```python
from build123d import *

# Parameters (mm, degrees)
IZIM1_R                     = 4
Y_KSEKLIK_EKSTR_ZYON1_DEPTH = 16
IZIM2_W                     = 25
IZIM2_H                     = 6
KES_EKSTR_ZYON1_DEPTH       = 35
KES_EKSTR_ZYON2_DEPTH       = 36
KES_EKSTR_ZYON2_DEPTH_BACK  = 20
IZIM3_R                     = 3
SKETCH2_W                   = 46.387108154
SKETCH2_H                   = 28.761742624
CUT_EXTRUDE1_DEPTH          = 2
FILLET1_R                   = 5


with BuildPart() as part:
    # Çizim1 → Yükseklik-Ekstrüzyon1 (new body)
    with BuildSketch(Plane.XY):
        Polygon((-12.5, 28), (-12.5, -7), (12.5, -7), (12.5, 28), (12.5, 53), (6, 53), (4.5, 53), (4.5, 33), (-4.5, 33), (-4.5, 53), (-6, 53), (-12.5, 53), align=None)
        with Locations((0, 21)):
            Circle(IZIM1_R, mode=Mode.SUBTRACT)
        Circle(IZIM1_R, mode=Mode.SUBTRACT)
    extrude(amount=Y_KSEKLIK_EKSTR_ZYON1_DEPTH)

    # Çizim2 → Kes-Ekstrüzyon1 (cut)
    with BuildSketch(Plane.XZ.offset(7)):
        with Locations((0, 8)):
            Rectangle(IZIM2_W, IZIM2_H)
    extrude(amount=-KES_EKSTR_ZYON1_DEPTH, mode=Mode.SUBTRACT)

    # Çizim3 → Kes-Ekstrüzyon2 (cut, two sides: drawn at the far end of the back side and taken through both)
    with BuildSketch(Plane.ZY.offset(-4.5).offset(-KES_EKSTR_ZYON2_DEPTH_BACK)):
        with Locations(Location((8, 43, 0), (0, 0, 180))):
            Circle(IZIM3_R)
    extrude(amount=KES_EKSTR_ZYON2_DEPTH + KES_EKSTR_ZYON2_DEPTH_BACK, mode=Mode.SUBTRACT)

    # Sketch2 → Cut-Extrude1 (cut)
    with BuildSketch(Plane(origin=(0, 53, 0), x_dir=(1, 0, 0), z_dir=(0, 1, 0))):
        with Locations((-0.016890664, -9.346912489)):
            Rectangle(SKETCH2_W, SKETCH2_H)
    extrude(amount=-CUT_EXTRUDE1_DEPTH, mode=Mode.SUBTRACT)

    # Fillet1
    fillet1_edges = [part.edges().sort_by_distance(p)[0] for p in [
        (8.5, 51, 16),
        (-8.5, 51, 16),
        (8.5, 51, 0),
        (-8.5, 51, 0),
    ]]
    fillet(fillet1_edges, radius=FILLET1_R)


solid = part.part
```
Geometry check sheet. Reference: the model listing, model coordinates, mm. A direction names the side the tool comes from. Give positions to 0.01 mm unless a question says otherwise; leave off trailing zeros. Write each loop counter-clockwise with the first axis right and the second up, starting at its lowest first coordinate (ties: lowest second). Pieces come first, ordered by that corner, then holes. Notation, with made-up numbers: (-21.75, 85) -> (8.25, 85) arc R18 cw to (8.25, 111) -> close; hole circle Ø9 at (16.5, 16). An arc over 180 degrees is marked (long way). Use one line per item in the form item = value.
Item 1: Depth check by flat-ended pin: pin 1 Ø1.8 at (x, z) = (0, 7.5) entering from -Y; pin 2 Ø5.5 at (y, z) = (43, 8) entering from +X; pin 3 Ø2.5 at (x, z) = (1, 11) entering from +Y. Enter the tip coordinate at first touch or a pass-through.
Results list:
pin_1 = 28
pin_2 = through
pin_3 = 33
Item 2: Sectioned sample at D-D on y = 6. Enter the section's corners in (x, z).
Results list:
outline = (-12.5, 0) -> (12.5, 0) -> (12.5, 5) -> (-12.5, 5) -> close; (-12.5, 11) -> (12.5, 11) -> (12.5, 16) -> (-12.5, 16) -> close
Item 3: Sectioned sample at A-A on x = 0. Enter the section's corners in (y, z).
Results list:
outline = (-7, 0) -> (-4, 0) -> (-4, 5) -> (-7, 5) -> close; (-7, 11) -> (-4, 11) -> (-4, 16) -> (-7, 16) -> close; (4, 0) -> (17, 0) -> (17, 5) -> (4, 5) -> close; (4, 11) -> (17, 11) -> (17, 16) -> (4, 16) -> close; (25, 0) -> (33, 0) -> (33, 16) -> (25, 16) -> (25, 11) -> (28, 11) -> (28, 5) -> (25, 5) -> close
Item 4: Access from +Z, -Z, +X, -X, +Y, -Y to the whole of each face (thin tool, end or side, straight path). Record for faces 4 (the cylindrical face through (-0.867, -3.905, 2.465)), 5 (the flat face through (0, 10, 11)), 6 (the flat face through (4.5, 40, 10)).
Results list:
face_4 = +Z, -Z
face_5 = +X, -X, -Y
face_6 = +Z, -Z, +Y
Item 5: Scan lines: line 1 (X direction, y = 43.5, z = 14); line 2 (Y direction, x = -9.75, z = 8); line 3 (Z direction, x = 8.5, y = 5). Record each from-to range of solid material in increasing order.
Results list:
line_1 = -12.5 to -4.5, 4.5 to 12.5
line_2 = 28 to 40, 46 to 51
line_3 = 0 to 5, 11 to 16
Item 6: Mould release check, pull along X, two halves, no side actions. Record for faces 1 (the flat face through (0, 33, 8)), 2 (the flat face through (0, 28, 8)), 3 (the flat face through (-12.5, 22.4, 11.4)): released by +X, released by -X, zero draft, split by the parting line, or undercut.
Results list:
face_1 = undercut
face_2 = zero draft
face_3 = released by -X
Item 7: Sectioned sample at C-C on z = 2. Enter the section's corners in (x, y).
Results list:
outline = (-12.5, -7) -> (12.5, -7) -> (12.5, 50) -> (4.5, 50) -> (4.5, 33) -> (-4.5, 33) -> (-4.5, 50) -> (-12.5, 50) -> close; hole circle Ø8 at (0, 0); hole circle Ø8 at (0, 21)
Item 8: Sectioned sample at B-B on y = 0. Enter the section's corners in (x, z), plus the area to 3 significant figures.
Results list:
outline = (-12.5, 0) -> (-4, 0) -> (-4, 5) -> (-12.5, 5) -> close; (-12.5, 11) -> (-4, 11) -> (-4, 16) -> (-12.5, 16) -> close; (4, 0) -> (12.5, 0) -> (12.5, 5) -> (4, 5) -> close; (4, 11) -> (12.5, 11) -> (12.5, 16) -> (4, 16) -> close
area = 170 mm2
